from build123d import *

# Parameters (mm, degrees)
SKETCH1_W           = 165
SKETCH1_H           = 110
BOSS_EXTRUDE1_DEPTH = 6
SKETCH2_W           = 5
SKETCH2_H           = 35
SKETCH2_W_2         = 74
SKETCH2_H_2         = 5
CUT_EXTRUDE1_DEPTH  = 3
SKETCH4_R           = 1.5
CUT_EXTRUDE2_DEPTH  = 111.956279878


with BuildPart() as part:
    # Sketch1 → Boss-Extrude1 (new body)
    with BuildSketch(Plane(origin=(0, 0, 0), x_dir=(1, 0, 0), z_dir=(0, 1, 0))):
        with Locations((-12.658730159, 1.746031746)):
            Rectangle(SKETCH1_W, SKETCH1_H)
    extrude(amount=BOSS_EXTRUDE1_DEPTH)

    # Sketch2 → Cut-Extrude1 (cut)
    with BuildSketch(Plane(origin=(0, 6, 0), x_dir=(1, 0, 0), z_dir=(0, 1, 0))):
        Polygon((-92.658730159, 48.746031746), (-92.658730159, 35.746031746), (-87.658730159, 35.746031746), (-87.658730159, 43.746031746), (-79.658730159, 43.746031746), (-79.658730159, 48.746031746), align=None)
        Polygon((-79.658730159, -40.253968254), (-79.658730159, -45.253968254), (-92.658730159, -45.253968254), (-92.658730159, -32.253968254), (-87.658730159, -32.253968254), (-87.658730159, -40.253968254), align=None)
        Polygon((54.341269841, 43.746031746), (54.341269841, 48.746031746), (67.341269841, 48.746031746), (67.341269841, 35.746031746), (62.341269841, 35.746031746), (62.341269841, 43.746031746), align=None)
        Polygon((62.341269841, -40.253968254), (54.341269841, -40.253968254), (54.341269841, -45.253968254), (67.341269841, -45.253968254), (67.341269841, -32.253968254), (62.341269841, -32.253968254), align=None)
        with Locations((64.841269841, 1.746031746)):
            Rectangle(SKETCH2_W, SKETCH2_H)
        with Locations((-90.158730159, 1.746031746)):
            Rectangle(SKETCH2_W, SKETCH2_H)
        with Locations((-12.658730159, -42.753968254)):
            Rectangle(SKETCH2_W_2, SKETCH2_H_2)
        with Locations((-12.658730159, 46.246031746)):
            Rectangle(SKETCH2_W_2, SKETCH2_H_2)
    extrude(amount=-CUT_EXTRUDE1_DEPTH, mode=Mode.SUBTRACT)

    # Sketch4 → Cut-Extrude2 (cut, through all)
    with BuildSketch(Plane(origin=(0, 6, 0), x_dir=(1, 0, 0), z_dir=(0, 1, 0))):
        with Locations(Location((-37.658730159, 38.746031746, 0), (0, 0, 270))):
            Circle(SKETCH4_R)
        with Locations(Location((12.341269841, 38.746031746, 0), (0, 0, 90))):
            Circle(SKETCH4_R)
        with Locations(Location((12.341269841, -35.253968254, 0), (0, 0, 270))):
            Circle(SKETCH4_R)
        with Locations(Location((-37.658730159, -35.253968254, 0), (0, 0, 90))):
            Circle(SKETCH4_R)
    extrude(amount=-CUT_EXTRUDE2_DEPTH, mode=Mode.SUBTRACT)


solid = part.part
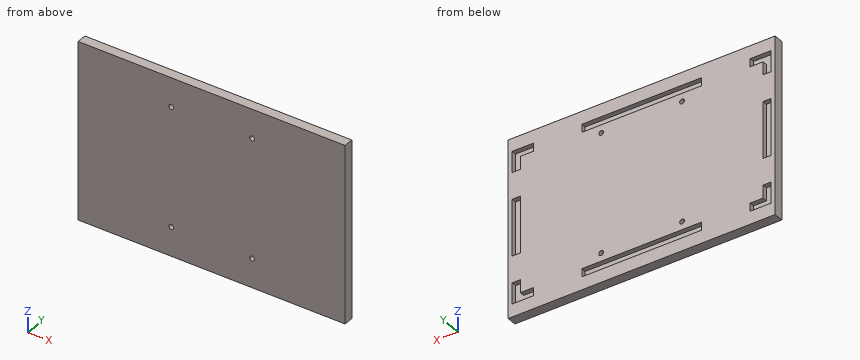
Source: CAD feature listing. Evaluate the final solid. Frame: model axes, mm. Give positions to 0.01 mm unless a question says otherwise; leave off trailing zeros. Order: outer loops, then holes, each group sorted by start corner. A loop starts at its lowest first (then second) coordinate and runs counter-clockwise, first axis right, second up. Notation, with made-up numbers: (57.5, 51.5) -> (85.5, 51.5) arc R16 cw to (85.5, 66.5) -> close; hole circle Ø10 at (-27.75, -12). An arc over 180 degrees is marked (long way). Write item = value, one per line.
Item 1: Section query A-A (x = -12). Output: boundary loops of the cut face in (y, z), then the cut area to 3 significant figures.
Check result:
outline = (0, -56.75) -> (6, -56.75) -> (6, -48.75) -> (3, -48.75) -> (3, -43.75) -> (6, -43.75) -> (6, 40.25) -> (3, 40.25) -> (3, 45.25) -> (6, 45.25) -> (6, 53.25) -> (0, 53.25) -> close
area = 630 mm²
Item 2: Section query C-C (y = 4.2). State how many separate pieces and enclosed holes the cut face has, then the cut area to 3 significant figures.
Check result:
separate_pieces = 1
enclosed_holes = 12
area = 16,600 mm²
Item 3: Ray query, probe 1 along Z at (x, y) = (62.5, 3.75); probe 2 along Z at (x, y) = (8, 4.3); probe 3 along X at (y, z) = (4.1, -47). Return the intervals inside material, ascending.
Check result:
probe_1 = -56.75 to -48.75, -35.75 to -19.25, 15.75 to 32.25, 45.25 to 53.25
probe_2 = -56.75 to -48.75, -43.75 to 40.25, 45.25 to 53.25
probe_3 = -95.16 to -92.66, -79.66 to -49.66, 24.34 to 54.34, 67.34 to 69.84
Item 4: Section query B-B (z = 4.5). Output: boundary loops of the cut face in (x, y), then the cut area to 3 significant figures.
Check result:
outline = (-95.16, 0) -> (69.84, 0) -> (69.84, 6) -> (67.34, 6) -> (67.34, 3) -> (62.34, 3) -> (62.34, 6) -> (-87.66, 6) -> (-87.66, 3) -> (-92.66, 3) -> (-92.66, 6) -> (-95.16, 6) -> close
area = 960 mm²
